```python
from build123d import *

# Parameters (mm, degrees)
SKETCH1_W           = 1100
SKETCH1_H           = 100
BOSS_EXTRUDE1_DEPTH = 34
SKETCH2_R           = 3
CUT_EXTRUDE1_DEPTH  = 554.313654269
LPATTERN1_COUNT     = 2
LPATTERN1_PITCH     = 440
CUT_EXTRUDE2_DEPTH  = 554.313654269
CUT_EXTRUDE3_DEPTH  = 554.313654269
CUT_EXTRUDE4_DEPTH  = 8


with BuildPart() as part:
    # Sketch1 → Boss-Extrude1 (new body)
    with BuildSketch(Plane(origin=(0, 0, 0), x_dir=(1, 0, 0), z_dir=(0, 1, 0))):
        Rectangle(SKETCH1_W, SKETCH1_H)
    extrude(amount=BOSS_EXTRUDE1_DEPTH)

    # Sketch2 → Cut-Extrude1 (cut, through all)
    with BuildSketch(Plane(origin=(0, 34, 0), x_dir=(1, 0, 0), z_dir=(0, 1, 0))):
        with Locations(Location((0, 0, 0), (0, 0, 270))):
            Circle(SKETCH2_R)
    cut_extrude1 = extrude(amount=-CUT_EXTRUDE1_DEPTH, mode=Mode.SUBTRACT)

    # LPattern1: Cut-Extrude1 ×2
    with Locations(*[(i * LPATTERN1_PITCH, 0, 0) for i in range(1, LPATTERN1_COUNT)]):
        add(cut_extrude1, mode=Mode.SUBTRACT)

    # Sketch3 → Cut-Extrude2 (cut, through all)
    with BuildSketch(Plane(origin=(0, 34, 0), x_dir=(1, 0, 0), z_dir=(0, 1, 0))):
        Polygon((540.762594459, 1.774699353), (414.907482272, 119.078541768), (523.885555732, 236.000949243), (780.808453445, 33.355832904), (490.286548009, -251.902570915), (394.883300151, -154.73897124), align=None)
    extrude(amount=-CUT_EXTRUDE2_DEPTH, mode=Mode.SUBTRACT)

    # Sketch4 → Cut-Extrude3 (cut, through all)
    with BuildSketch(Plane.XZ):
        Polygon((-439.548903775, -50), (-521.367085593, 37.782601488), (-461.555021583, 93.530713814), (-639.566149279, 284.518579051), (-887.964366722, 45.983956755), (-622.18599326, -220.227748335), align=None)
    extrude(amount=-CUT_EXTRUDE3_DEPTH, mode=Mode.SUBTRACT)

    # Sketch5 → Cut-Extrude4 (cut)
    with BuildSketch(Plane.XZ):
        Polygon((457.65907548, -125.279728267), (196.673608083, 154.731178471), (458.273207913, 338.877030437), (810.658904172, -71.072769519), align=None)
    extrude(amount=-CUT_EXTRUDE4_DEPTH, mode=Mode.SUBTRACT)


solid = part.part
```
Build history of the part. All positions in model axes, mm. A direction names the side the tool comes from. Round coordinates to 2 decimals unless told otherwise and drop trailing zeros. Loops run counter-clockwise (first coordinate to the right, second up) from the corner with the lowest first, then second, coordinate; pieces in that order, holes last.
Item 1: Which spindle directions (+Z, -Z, +X, -X, +Y, -Y) get a long thin tool onto all of the face, cutting with end or side? Do faces 1 (the face through (419, 8, 1)), 2 (the face through (2, 34, 10)). Say none if no direction does.
Item 2: Pin check, flat tips, straight feed: P1, Ø5, axis at x = 0, z = 0, coming from the -Y side; P2, Ø8, axis at y = 10.5, z = -16.5, coming from the -X side; P3, Ø12, axis at y = 23.5, z = 3, coming from the +X side; P4, Ø1, axis at y = 4, z = 10, coming from the +X side. Stop position of each tip, or through.
Item 3: Drill centre lines: line 1 along Z through (x, y) = (440, 21.75); line 2 along X through (y, z) = (17.5, 0); line 3 along Y through (x, z) = (427.5, 44). Where is each one in solid material? Low to high.
Item 4: Saw through at C-C (x = 374.5). List the corners of the cut face in (y, z).
Item 5: Saw through at A-A (y = 14). List the corners of the cut face in (x, z).
Item 6: Saw through at B-B (z = 28). List the corners of the cut face in (x, y), then the cut area to 3 significant figures.
Worked answers:
1. face 1: +Z, +X, -Y
1. face 2: +Z, -Z, +X, -X, +Y
2. P1: passes through
2. P2: stops at x = -474.5
2. P3: stops at x = 540.76
2. P4: stops at x = 332.04
3. line 1: z = -50 to -3, 3 to 50
3. line 2: x = -486.15 to -3, 3 to 437, 443 to 539.11
3. line 3: y = 8 to 34
4. outline: (0, -50) - (34, -50) - (34, 50) - (8, 50) - (8, -36.06) - (0, -36.06) - close
5. outline: (-521.37, 37.78) - (-439.55, -50) - (489.02, -50) - (540.76, -1.77) - (492.51, 50) - (-508.26, 50) - close; hole circle Ø6 at (0, 0); hole circle Ø6 at (440, 0)
6. outline: (-512.25, 0) - (314.79, 0) - (314.79, 8) - (513.01, 8) - (513.01, 34) - (-512.25, 34) - close
6. area: 33,300 mm2
